Could you check a few things on this model? Use its own coordinates, in mm. Face numbers are marked on the shaded views. A direction names the side the tool comes from. Give positions to 0.01 mm unless a question says otherwise; leave off trailing zeros. Loops run counter-clockwise (first coordinate to the right, second up) from the corner with the lowest first, then second, coordinate; pieces in that order, holes last. Notation, with made-up numbers: (70.25, -34) - (92.25, -34) arc R28 ccw to (92.25, -3) - close; hole circle Ø5 at (43, 60). An arc over 180 degrees is marked (long way). Write each question's results on one line, items separated by ' | '. Start each with the question number.
1) On a 3-axis mill with a long thin cutter (end or side, diameter ignored), from which of +Z, -Z, +X, -X, +Y, -Y can I reach the whole of each face in a straight line? I mean the marked faces 4, 5, 6 and 7. Say none if no direction works.
2) I want a section at B-B, the plane z = 6.75. Write out the boundary of the cut face in (x, y), and give its area (3 significant figures).
3) I want a section at A-A, the plane x = 0. Write out the boundary of the cut face in (y, z), and give its area (3 significant figures).
4) If we mould it in two halves opening along X, with no side actions, what happens to the marked faces 1, 2 and 3? For each: +X half, -X half, draft (parallel to the pull), parting line (faces both ways), or undercut.
5) If I drill on probe 1 along Y at (x, z) = (0, 6.25); probe 2 along X at (y, z) = (27, 10.25); probe 3 along Y at (x, z) = (-12.5, 13.5), over which ranges is the centre line in solid material (lowest first)? Write a range as [from, to].
6) I'm going to push flat-ended pins straight in: pin 1 (1 mm diameter, centred on x = 0, z = 3.5, fed in from +Y); pin 2 (1.5 mm diameter, centred on x = 6.5, z = 9.5, fed in from -Y); pin 3 (4 mm diameter, centred on x = -11, y = 24.5, fed in from +Z). Where does each tip first touch, or does it pass through?
7) I want a section at D-D, the plane x = -6.5. Write out the boundary of the cut face in (y, z), and give its area (3 significant figures).
8) I want a section at C-C, the plane y = 7. Write out the boundary of the cut face in (x, z).
from build123d import *

# Parameters (mm, degrees)
ESQUISSE1_R             = 10
ESQUISSE1_R_2           = 4
BASE_EXTRUSION_DEPTH    = 20
CONG_1_R                = 4
ESQUISSE4_W             = 14
ESQUISSE4_H             = 23
ENL_V_MAT_EXTRU_4_DEPTH = 10


with BuildPart() as part:
    # Esquisse1 → Base-Extrusion (new body)
    with BuildSketch(Plane.XY):
        with BuildLine():
            Line((10, 27), (10, 12.489995997))
            ThreePointArc((10, 12.489995997), (0, -16), (-10, 12.489995997))
            Line((-10, 12.489995997), (-10, 27))
            ThreePointArc((-10, 27), (0, 37), (10, 27))
        make_face()
        Circle(ESQUISSE1_R, mode=Mode.SUBTRACT)
        with Locations((0, 27)):
            Circle(ESQUISSE1_R_2, mode=Mode.SUBTRACT)
    extrude(amount=BASE_EXTRUSION_DEPTH)

    # Congé1
    cong_1_edges = [part.edges().sort_by_distance(p)[0] for p in [
        (10, 12.489995997, 10),
        (-10, 12.489995997, 10),
    ]]
    fillet(cong_1_edges, radius=CONG_1_R)

    # Esquisse4 → Enlèv. mat.-Extru.4 (cut, symmetric)
    with BuildSketch(Plane(origin=(0, 0, 0), x_dir=(0, 0, -1), z_dir=(1, 0, 0))):
        with Locations((-21, 26.5)):
            Rectangle(ESQUISSE4_W, ESQUISSE4_H)
        with Locations((1, 26.5)):
            Rectangle(ESQUISSE4_W, ESQUISSE4_H)
    extrude(amount=ENL_V_MAT_EXTRU_4_DEPTH, both=True, mode=Mode.SUBTRACT)


solid = part.part
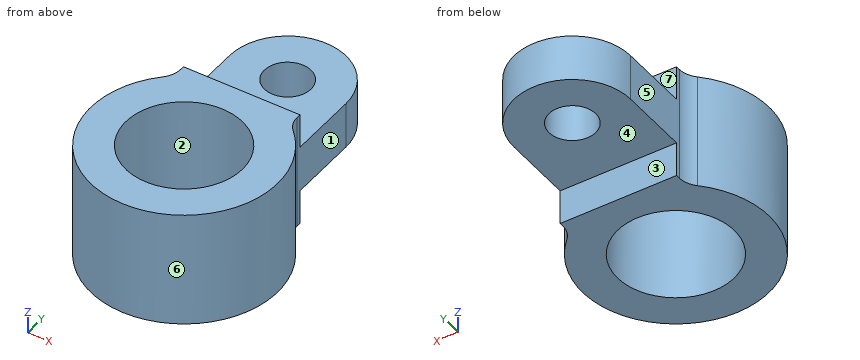
Answers:
1) face 4: -Z, +X, -X, +Y | face 5: +Z, -Z, -X, +Y | face 6: +Z, -Z | face 7: +Z, +X, -X, +Y
2) outline: (-11.2, 11.43) arc R16 ccw (long way) to (11.2, 11.43) arc R4 cw to (10, 14.28) - (10, 27) arc R10 ccw to (-10, 27) - (-10, 14.28) arc R4 cw to start; hole circle Ø20 at (0, 0); hole circle Ø8 at (0, 27) | area: 840 mm2
3) outline: (-16, 0) - (-10, 0) - (-10, 20) - (-16, 20) - close; (10, 0) - (15, 0) - (15, 6) - (23, 6) - (23, 14) - (15, 14) - (15, 20) - (10, 20) - close; (31, 6) - (37, 6) - (37, 14) - (31, 14) - close | area: 332 mm2
4) face 1: +X half | face 2: undercut | face 3: draft
5) probe 1: y = [-16, -10], [10, 23], [31, 37] | probe 2: x = [-10, -4], [4, 10] | probe 3: y = [-9.99, 9.99]
6) pin 1: stops at y = 15 | pin 2: stops at y = -14.93 | pin 3: stops at z = 14
7) outline: (-14.62, 0) - (-7.6, 0) - (-7.6, 20) - (-14.62, 20) - close; (7.6, 0) - (15, 0) - (15, 6) - (34.6, 6) - (34.6, 14) - (15, 14) - (15, 20) - (7.6, 20) - close | area: 445 mm2
8) outline: (-14.39, 0) - (-7.14, 0) - (-7.14, 20) - (-14.39, 20) - close; (7.14, 0) - (14.39, 0) - (14.39, 20) - (7.14, 20) - close
